Geometry check sheet. Reference: the model listing, model coordinates, mm. Face numbers are marked on the shaded views. A direction names the side the tool comes from. Give positions to 0.01 mm unless a question says otherwise; leave off trailing zeros. Write each loop counter-clockwise with the first axis right and the second up, starting at its lowest first coordinate (ties: lowest second). Pieces come first, ordered by that corner, then holes.
(1) Cross-section at D-D (x = 4.5). Record the boundary of the cut face in (y, z), and give its area (3 significant figures).
(2) Mould release check, pull along Y, two halves, no side actions. Record for the marked faces 1, 2, 3 and 4: +Y half, -Y half, draft (parallel to the pull), parting line (faces both ways), or undercut.
(3) Thickness scan on line 1 along X through (y, z) = (-9.5, -1.5); line 2 along X through (y, z) = (13, -0.2); line 3 along Y through (x, z) = (2.25, -0.75). Record the ranges inside material, lowest first.
(4) Depth check by flat-ended pin: P1, Ø6, axis at x = -2.5, y = 3, coming from the +Z side. Enter the tip coordinate at first touch or a pass-through.
(5) Cross-section at A-A (y = 1.5). Record the boundary of the cut face in (x, z).
(6) Tool access check on the marked faces 5 and 6. Record the directions out of +Z, -Z, +X, -X, +Y, -Y that give a thin tool (end or side, any length) a straight path to the whole face; none if there is none.
(7) Cross-section at C-C (x = 2). Record the boundary of the cut face in (y, z), and give its area (3 significant figures).
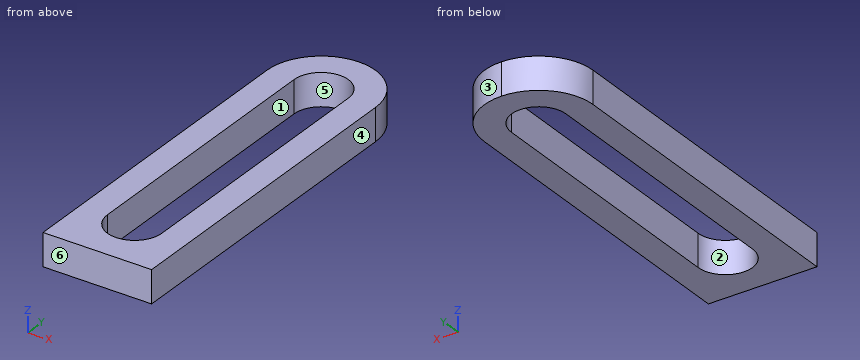
```python
from build123d import *

# Parameters (mm, degrees)
SKETCH1_W          = 10
SKETCH1_H          = 35
BASE_FLANGE1_DEPTH = 3
FILLET1_R          = 5


# Sheet-metal steps are written as plain solids
with BuildPart() as part:
    # Sketch1 → Base-Flange1 (new body)
    with BuildSketch(Plane.XY):
        Rectangle(SKETCH1_W, SKETCH1_H)
        with BuildLine():
            Line((-2.5, -12.5), (-2.5, 12.5))
            ThreePointArc((-2.5, 12.5), (0, 15), (2.5, 12.5))
            Line((2.5, 12.5), (2.5, -12.5))
            ThreePointArc((2.5, -12.5), (0, -15), (-2.5, -12.5))
        make_face(mode=Mode.SUBTRACT)
    extrude(amount=-BASE_FLANGE1_DEPTH)

    # Fillet1
    fillet1_edges = [part.edges().sort_by_distance(p)[0] for p in [
        (-5, 17.5, -1.5),
        (5, 17.5, -1.5),
    ]]
    fillet(fillet1_edges, radius=FILLET1_R - 0.0001)  # a hair under: the kernel refuses the full size


solid = part.part
```
Reply:
1. outline: (-17.5, -3) - (14.68, -3) - (14.68, 0) - (-17.5, 0) - close
1. area: 96.5 mm2
2. face 1: undercut
2. face 2: undercut
2. face 3: +Y half
2. face 4: draft
3. line 1: x = -5 to -2.5, 2.5 to 5
3. line 2: x = -4.97 to -2.45, 2.45 to 4.97
3. line 3: y = -17.5 to -13.59, 13.59 to 16.97
4. P1: stops at z = 0
5. outline: (-5, -3) - (-2.5, -3) - (-2.5, 0) - (-5, 0) - close; (2.5, -3) - (5, -3) - (5, 0) - (2.5, 0) - close
6. face 5: +Z, -Z
6. face 6: +Z, -Z, +X, -X, -Y
7. outline: (-17.5, -3) - (-14, -3) - (-14, 0) - (-17.5, 0) - close; (14, -3) - (17.08, -3) - (17.08, 0) - (14, 0) - close
7. area: 19.7 mm2
